Source: CAD feature listing. Evaluate the final solid. Frame: model axes, mm. Face numbers are marked on the shaded views. Round coordinates to 2 decimals unless told otherwise and drop trailing zeros. Write each loop counter-clockwise with the first axis right and the second up, starting at its lowest first coordinate (ties: lowest second). Pieces come first, ordered by that corner, then holes. Notation, with made-up numbers: (-5, 44) -> (41, 44) arc R18 cw to (41, 48) -> close; hole circle Ø4 at (77, -32.75). An arc over 180 degrees is marked (long way). Put each result on its own line as item: value.
```python
from build123d import *

# Parameters (mm, degrees)
F0_R     = 11
F1_DEPTH = 6.35
F2_R     = 2


with BuildPart() as f1:
    # F0 (on Top) → F1 (new body)
    with BuildSketch(Plane.XY):
        with BuildLine():
            ThreePointArc((-28.195265, -0.164368), (-38.373827, 5.331046), (-41.929181, 16.338414))
            ThreePointArc((-41.929181, 16.338414), (-38.971143, -22.5), (-6.815109, -44.480943))
            ThreePointArc((-6.815109, -44.480943), (-14.570092, -35.898232), (-14.23998, -24.335632))
            ThreePointArc((-14.23998, -24.335632), (0, -15), (14.23998, -24.335632))
            ThreePointArc((14.23998, -24.335632), (14.570092, -35.898232), (6.815109, -44.480943))
            ThreePointArc((6.815109, -44.480943), (38.971143, -22.5), (41.929181, 16.338414))
            ThreePointArc((41.929181, 16.338414), (38.373827, 5.331046), (28.195265, -0.164368))
            ThreePointArc((28.195265, -0.164368), (12.990381, 7.5), (13.955286, 24.5))
            ThreePointArc((13.955286, 24.5), (23.803735, 30.567186), (35.114072, 28.142529))
            ThreePointArc((35.114072, 28.142529), (0, 45), (-35.114072, 28.142529))
            ThreePointArc((-35.114072, 28.142529), (-23.803735, 30.567186), (-13.955286, 24.5))
            ThreePointArc((-13.955286, 24.5), (-12.990381, 7.5), (-28.195265, -0.164368))
        make_face()
        with Locations((-25.980762, -15)):
            Circle(F0_R, mode=Mode.SUBTRACT)
        Circle(F0_R, mode=Mode.SUBTRACT)
        with Locations((25.980762, -15)):
            Circle(F0_R, mode=Mode.SUBTRACT)
        with Locations((0, 30)):
            Circle(F0_R, mode=Mode.SUBTRACT)
    extrude(amount=F1_DEPTH)

    # F2
    f2_edges = [f1.edges().sort_by_distance(p)[0] for p in [
        (6.815109, -44.480943, 3.175),
        (-6.815109, -44.480943, 3.175),
        (-41.929181, 16.338414, 3.175),
        (-35.114072, 28.142529, 3.175),
        (35.114072, 28.142529, 3.175),
        (41.929181, 16.338414, 3.175),
    ]]
    fillet(f2_edges, radius=F2_R)


solid = f1.part
```
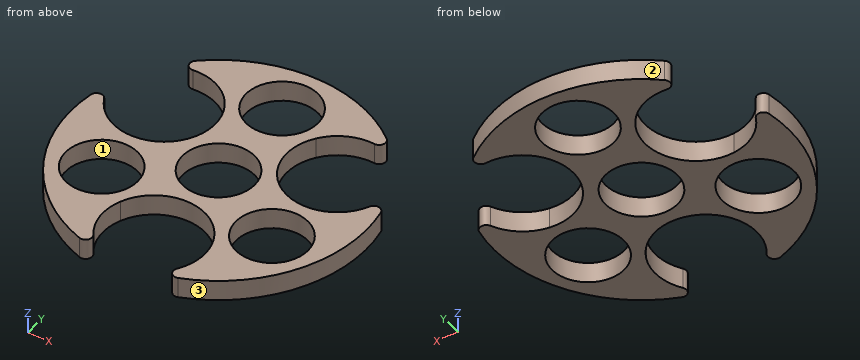
Q1. Draft query along X for the marked faces 1, 2 and 3. Return one class per face: +X half, -X half, draft (parallel to the pull), parting line (faces both ways), or undercut.
Ans:
face 1: undercut
face 2: parting line
face 3: +X half
Q2. Cut plane A-A on x = -33. Output: boundary loops of the cut face in (y, z), and give its area (3 significant figures).
Ans:
outline: (-30.59, 0) -> (-23.47, 0) -> (-23.47, 6.35) -> (-30.59, 6.35) -> close; (-6.53, 0) -> (1.19, 0) -> (1.19, 6.35) -> (-6.53, 6.35) -> close
area: 94.3 mm^2
Q3. Material intervals for line 1 (Y direction, x = 0, z = 4.5); line 2 (Y direction, x = -24, z = 0.75); line 3 (X direction, y = -20, z = 3.5), sorted ascending. Write a range as [from, to].
Ans:
line 1: y = [-15, -11], [11, 19], [41, 45]
line 2: y = [-38.07, -25.82], [-4.18, -0.07], [30.6, 38.07]
line 3: x = [-40.31, -35.78], [-16.18, -11.41], [11.41, 16.18], [35.78, 40.31]
Q4. Pin query (flat end, axial travel): pin 1 (1.5 mm diameter, centred on y = -25, z = 2.5, fed in from +X); pin 2 (17.5 mm diameter, centred on x = 0, y = 30, fed in from -Z). Return the tip coordinate at first contact, or that it passes through.
Ans:
pin 1: stops at x = 37.91
pin 2: passes through
Q5. Cut plane D-D on x = 4. Output: boundary loops of the cut face in (y, z), and give its area (3 significant figures).
Ans:
outline: (-15.52, 0) -> (-10.25, 0) -> (-10.25, 6.35) -> (-15.52, 6.35) -> close; (10.25, 0) -> (19.75, 0) -> (19.75, 6.35) -> (10.25, 6.35) -> close; (40.25, 0) -> (44.82, 0) -> (44.82, 6.35) -> (40.25, 6.35) -> close
area: 123 mm^2
Q6. Cut plane B-B on x = -18. Output: boundary loops of the cut face in (y, z).
Ans:
outline: (-41.24, 0) -> (-22.57, 0) -> (-22.57, 6.35) -> (-41.24, 6.35) -> close; (-7.43, 0) -> (2.23, 0) -> (2.23, 6.35) -> (-7.43, 6.35) -> close; (28.3, 0) -> (41.24, 0) -> (41.24, 6.35) -> (28.3, 6.35) -> close
Q7. Cut plane C-C on y = 21.5. Output: boundary loops of the cut face in (x, z).
Ans:
outline: (-12.22, 0) -> (-6.98, 0) -> (-6.98, 6.35) -> (-12.22, 6.35) -> close; (6.98, 0) -> (12.22, 0) -> (12.22, 6.35) -> (6.98, 6.35) -> close
